Geometry: final body of the model. Coordinates: model frame, mm. Round coordinates to 2 decimals unless told otherwise and drop trailing zeros. Loops run counter-clockwise (first coordinate to the right, second up) from the corner with the lowest first, then second, coordinate; pieces in that order, holes last. Notation, with made-up numbers: (31, 37.25) - (74, 37.25) arc R23 cw to (74, 67.25) - close; hole circle Ø5 at (-2.5, 58.5). An arc over 180 degrees is marked (long way). Answer as CSV lines item,"result".
from build123d import *

# Parameters (mm, degrees)
SKETCH003_R   = 138.5
SKETCH003_R_2 = 11
PAD002_DEPTH  = 30
SKETCH004_R   = 95
PAD003_DEPTH  = 55
SKETCH005_R   = 84.1375
POCKET_DEPTH  = 85.001


with BuildPart() as part:
    # Sketch003 → Pad002 (new body)
    with BuildSketch(Plane.XZ.offset(-3)):
        Circle(SKETCH003_R)
        with Locations((-120, 0)):
            Circle(SKETCH003_R_2, mode=Mode.SUBTRACT)
        with Locations((-84.852814, 84.852814)):
            Circle(SKETCH003_R_2, mode=Mode.SUBTRACT)
        with Locations((0, 120)):
            Circle(SKETCH003_R_2, mode=Mode.SUBTRACT)
        with Locations((84.852814, 84.852814)):
            Circle(SKETCH003_R_2, mode=Mode.SUBTRACT)
        with Locations((120, 0)):
            Circle(SKETCH003_R_2, mode=Mode.SUBTRACT)
        with Locations((84.852814, -84.852814)):
            Circle(SKETCH003_R_2, mode=Mode.SUBTRACT)
        with Locations((0, -120)):
            Circle(SKETCH003_R_2, mode=Mode.SUBTRACT)
        with Locations((-84.852814, -84.852814)):
            Circle(SKETCH003_R_2, mode=Mode.SUBTRACT)
    extrude(amount=-PAD002_DEPTH)

    # Sketch004 (on Face11 of Pad002) → Pad003 (join)
    with BuildSketch(Plane(origin=(0, 33, 0), x_dir=(1, 0, 0), z_dir=(0, 1, 0))):
        Circle(SKETCH004_R)
    extrude(amount=PAD003_DEPTH)

    # Sketch005 (on Face13 of Pad003) → Pocket (cut, through all)
    with BuildSketch(Plane(origin=(0, 88, 0), x_dir=(1, 0, 0), z_dir=(0, 1, 0))):
        Circle(SKETCH005_R)
    extrude(amount=-POCKET_DEPTH, mode=Mode.SUBTRACT)


solid = part.part
(1) Section A-A (x = 0). Output: boundary loops of the cut face in (y, z), and give its area (3 significant figures).
Findings below:
outline,"(3, -138.5) - (33, -138.5) - (33, -131) - (3, -131) - close; (3, -109) - (33, -109) - (33, -95) - (88, -95) - (88, -84.14) - (3, -84.14) - close; (3, 84.14) - (88, 84.14) - (88, 95) - (33, 95) - (33, 109) - (3, 109) - close; (3, 131) - (33, 131) - (33, 138.5) - (3, 138.5) - close"
area,"3,140 mm2"
(2) Section D-D (y = 45.5). Output: boundary loops of the cut face in (x, z) (1 decimal).
Findings below:
outline,"circle Ø190 at (0, 0); hole circle Ø168.3 at (0, 0)"
(3) Section B-B (z = 0). Output: boundary loops of the cut face in (x, y).
Findings below:
outline,"(-138.5, 3) - (-131, 3) - (-131, 33) - (-138.5, 33) - close; (-109, 3) - (-84.14, 3) - (-84.14, 88) - (-95, 88) - (-95, 33) - (-109, 33) - close; (84.14, 3) - (109, 3) - (109, 33) - (95, 33) - (95, 88) - (84.14, 88) - close; (131, 3) - (138.5, 3) - (138.5, 33) - (131, 33) - close"
(4) Pin query (flat end, axial travel): P1, Ø1, axis at x = -48, y = 71.5, coming from the +Z side; P2, Ø2, axis at x = -54.5, y = 33, coming from the -Z side; P3, Ø13, axis at x = -120, z = 0, coming from the -Y side; P4, Ø1.5, axis at x = -23.5, y = 12.5, coming from the +Z side. Return the tip coordinate at first contact, or that it passes through.
Findings below:
P1,"z = 82.27"
P2,"z = -127.75"
P3,"through"
P4,"z = 136.62"
(5) Draft query along Z for faces 1 (the face through (-20.59, 60.11, 92.74)), 2 (the face through (30, 33, -92)), 3 (the face through (-1.432, 17.79, 130.906)), 4 (the face through (83.421, 17.79, -73.946)). Return one class per face: pulls with the +Z half, pulls with the -Z half, needs draft (parallel to the pull), parting line crosses it, or undercut.
Findings below:
face 1,"parting line crosses it"
face 2,"needs draft"
face 3,"undercut"
face 4,"undercut"
(6) Section C-C (z = -120). Output: boundary loops of the cut face in (x, y), and give its area (3 significant figures).
Findings below:
outline,"(-69.15, 3) - (-11, 3) - (-11, 33) - (-69.15, 33) - close; (11, 3) - (69.15, 3) - (69.15, 33) - (11, 33) - close"
area,"3,490 mm2"
(7) Material intervals for line 1 along Z through (x, y) = (0, 37); line 2 along Z through (x, y) = (0, 25.25), sorted ascending.
Findings below:
line 1,"-95 to -84.14, 84.14 to 95"
line 2,"-138.5 to -131, -109 to -84.14, 84.14 to 109, 131 to 138.5"
